Check sheet for the drawn part. Datum: minimum x, y, z corner. Units: mm. A direction names the side the tool comes from. Round coordinates to 2 decimals unless told otherwise and drop trailing zeros. Write each loop counter-clockwise with the first axis right and the second up, starting at its lowest first coordinate (ties: lowest second). Pieces come first, ordered by that corner, then holes. Notation, with made-up numbers: (29.5, -5) -> (86.5, -5) arc R14 cw to (86.5, 4) -> close; hole circle Ø5 at (0, 80.5). An arc over 180 degrees is marked (long way). One line per item, written item: value. Start each with the question number.
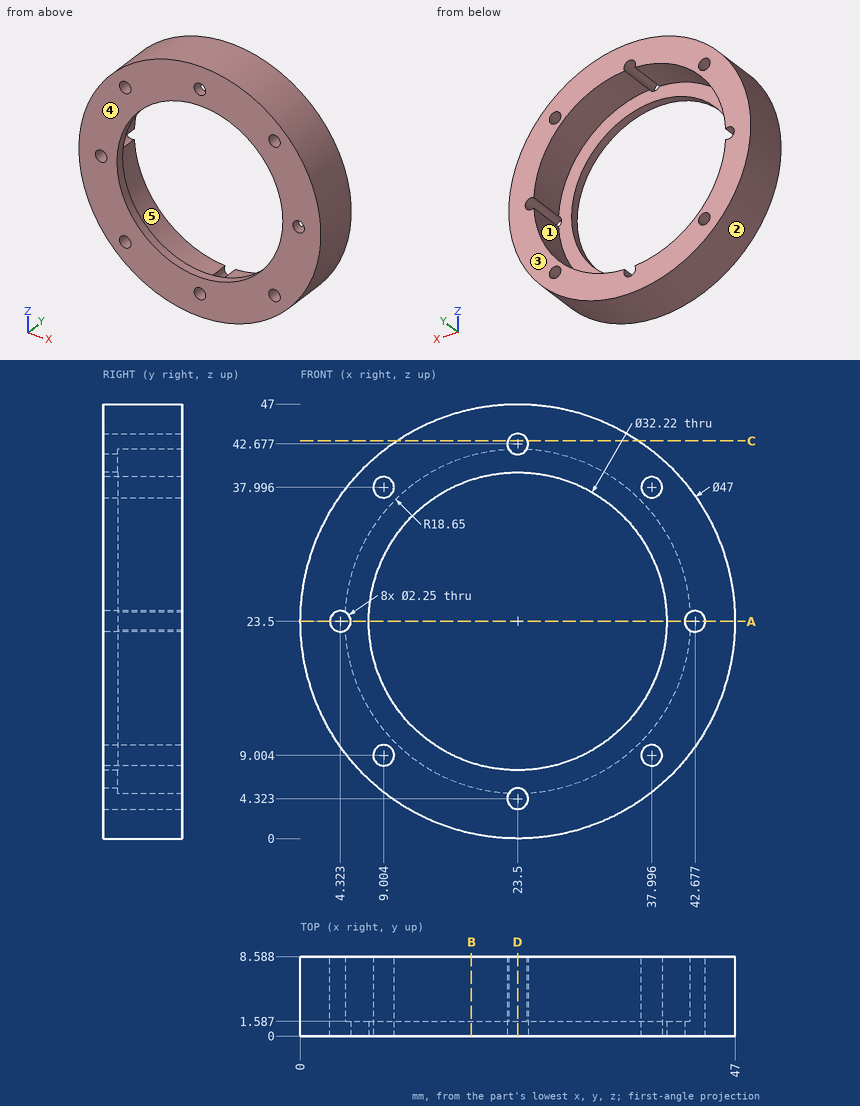
1. Access from +Z, -Z, +X, -X, +Y, -Y to the whole of each face (thin tool, end or side, straight path). Record for the marked faces 4 and 5.
2. Release check for a two-part mould opening along X. For the marked faces 1, 2 and 3 record: +X half, -X half, draft (parallel to the pull), parting line (faces both ways), or undercut.
3. Cross-section at B-B (x = 18.5). Record the cut outline in (y, z) (1 decimal).
4. Material ranges on probe 1 along X at (y, z) = (5, 39) (1 decimal); probe 2 along X at (y, z) = (2, 9.5) (1 decimal); probe 3 along Z at (x, y) = (8.5, 6) (1 decimal), recorded low to high.
5. Cross-section at A-A (z = 23.5). Record the cut outline in (x, y).
6. Depth check by flat-ended pin: pin 1 Ø2 at (x, z) = (7.5, 26) entering from +Y; pin 2 Ø2 at (y, z) = (2, 7) entering from +X (1 decimal). Enter the tip coordinate at first touch or a pass-through.
7. Cross-section at D-D (x = 23.5). Record the cut outline in (y, z).
8. Cross-section at C-C (z = 43). Record the cut outline in (x, y) (1 decimal), plus the area to 3 significant figures.
Working result:
1. face 4: +Z, -Z, +X, -X, -Y
1. face 5: +Y
2. face 1: undercut
2. face 2: parting line
2. face 3: draft
3. outline: (0, 0.5) -> (8.6, 0.5) -> (8.6, 5.5) -> (1.6, 5.5) -> (1.6, 8.2) -> (0, 8.2) -> close; (0, 38.8) -> (1.6, 38.8) -> (1.6, 41.5) -> (8.6, 41.5) -> (8.6, 46.5) -> (0, 46.5) -> close
4. probe 1: x = 5.8 to 8.5, 9.5 to 13.1, 33.9 to 37.5, 38.5 to 41.2
4. probe 2: x = 4.6 to 8, 10 to 11.2, 35.8 to 37, 39 to 42.4
4. probe 3: z = 5.4 to 8, 10 to 12.4, 34.6 to 37, 39 to 41.6
5. outline: (0, 0) -> (3.2, 0) -> (3.2, 8.59) -> (0, 8.59) -> close; (5.45, 0) -> (7.39, 0) -> (7.39, 1.59) -> (5.45, 1.59) -> close; (39.61, 0) -> (41.55, 0) -> (41.55, 1.59) -> (39.61, 1.59) -> close; (43.8, 0) -> (47, 0) -> (47, 8.59) -> (43.8, 8.59) -> close
6. pin 1: stops at y = 1.59
6. pin 2: stops at x = 41.2
7. outline: (0, 0) -> (8.59, 0) -> (8.59, 3.2) -> (0, 3.2) -> close; (0, 5.45) -> (1.59, 5.45) -> (1.59, 7.39) -> (0, 7.39) -> close; (0, 39.61) -> (1.59, 39.61) -> (1.59, 41.55) -> (0, 41.55) -> close; (0, 43.8) -> (8.59, 43.8) -> (8.59, 47) -> (0, 47) -> close
8. outline: (10.4, 0) -> (22.4, 0) -> (22.4, 8.6) -> (10.4, 8.6) -> close; (24.6, 0) -> (36.6, 0) -> (36.6, 8.6) -> (24.6, 8.6) -> close
8. area: 207 mm^2
